from build123d import *

# Parameters (mm, degrees)
F1_DEPTH = 85
F3_DEPTH = 45
F5_DEPTH = 30
F6_SIZE2 = 20
F6_SIZE  = 68
F8_DEPTH = 30
F9_SIZE2 = 22
F9_SIZE  = 88


with BuildPart() as f1:
    # F0 (on Front) → F1 (new body)
    with BuildSketch(Plane.XZ):
        Polygon((-22.5, 0), (0, 0), (0, 2007.5), (785, 2007.5), (785, 0), (807.5, 0), (807.5, 2030), (-22.5, 2030), align=None)
    extrude(amount=F1_DEPTH)

    # F2 (on face) → F3 (join)
    with BuildSketch(Plane(origin=(0, 0, 0), x_dir=(-1, 0, 0), z_dir=(0, 1, 0))):
        Polygon((12.5, 0), (22.5, 0), (32.5, 0), (32.5, 2040), (-817.5, 2040), (-817.5, 0), (-807.5, 0), (-797.5, 0), (-797.5, 2020), (12.5, 2020), align=None)
    extrude(amount=F3_DEPTH)

    # F4 (on face) → F5 (join)
    with BuildSketch(Plane(origin=(0, 45, 0), x_dir=(-1, 0, 0), z_dir=(0, 1, 0))):
        Polygon((-897.5, 0), (-817.5, 0), (-807.5, 0), (-807.5, 2035), (27.5, 2035), (27.5, 0), (32.5, 0), (112.5, 0), (112.5, 2120), (-897.5, 2120), align=None)
    extrude(amount=F5_DEPTH)

    # F6
    f6_edges = [f1.edges().sort_by_distance(p)[0] for p in [
        (390, 75, 2035),
        (-27.5, 75, 1017.5),
        (807.5, 75, 1017.5),
    ]]
    f6_side = f1.faces().sort_by_distance((852.5, 75, 23.482973))[0]
    chamfer(f6_edges, length=F6_SIZE, length2=F6_SIZE2, reference=f6_side)

    # F7 (on face) → F8 (join)
    with BuildSketch(Plane.XZ.offset(85)):
        Polygon((-118, 0), (-8, 0), (-8, 2015.5), (793, 2015.5), (793, 0), (903, 0), (903, 2125.5), (-118, 2125.5), align=None)
    extrude(amount=F8_DEPTH)

    # F9
    f9_edges = [f1.edges().sort_by_distance(p)[0] for p in [
        (793, -115, 1007.75),
        (392.5, -115, 2015.5),
        (-8, -115, 1007.75),
    ]]
    f9_side = f1.faces().sort_by_distance((-63, -115, 23.580058))[0]
    chamfer(f9_edges, length=F9_SIZE, length2=F9_SIZE2, reference=f9_side)


solid = f1.part
Verification items for the finished model (mm, model axes). A direction names the side the tool comes from. Round coordinates to 2 decimals unless told otherwise and drop trailing zeros. Loops run counter-clockwise (first coordinate to the right, second up) from the corner with the lowest first, then second, coordinate; pieces in that order, holes last. Notation, with made-up numbers: (51, 32) - (60, 32) arc R15 ccw to (60, 47) - close; hole circle Ø10 at (-23, -22.75). An arc over 180 degrees is marked (long way). Write item = value, one per line.
Q1. Sectioned sample at B-B on x = 416. Record the boundary of the cut face in (y, z).
Here are the results:
outline = (-115, 2103.5) - (-93, 2015.5) - (-85, 2015.5) - (-85, 2007.5) - (0, 2007.5) - (0, 2020) - (45, 2020) - (45, 2035) - (55, 2035) - (75, 2103) - (75, 2120) - (45, 2120) - (45, 2040) - (0, 2040) - (0, 2030) - (-85, 2030) - (-85, 2125.5) - (-115, 2125.5) - close
Q2. Tool access check on faces 5 (the flat face through (844, 45, 1222)), 6 (the flat face through (387, -42, 2007.5)), 7 (the flat face through (-51.384, -103.846, 1037.026)), 8 (the flat face through (397, 65, 2069)), 9 (the flat face through (807.5, -42, 1001)). Record the directions out of +Z, -Z, +X, -X, +Y, -Y that give a thin tool (end or side, any length) a straight path to the whole face; none if there is none.
Here are the results:
face_5 = +Z
face_6 = -Z, +Y, -Y
face_7 = -Z, -Y
face_8 = -Z, +Y
face_9 = +Z, -Z, +X
Q3. Depth check by flat-ended pin: pin 1 (2 mm diameter, centred on x = 127, y = 26, fed in from +Z); pin 2 (6 mm diameter, centred on x = 28.5, y = -89.5, fed in from -Z); pin 3 (1 mm diameter, centred on y = -59, z = 251, fed in from +X). Enter the tip coordinate at first touch or a pass-through.
Here are the results:
pin_1 = 2040
pin_2 = 2015.5
pin_3 = 807.5
Q4. Material ranges on L1, parallel to X at y = -11, z = 2004.5; L2, parallel to X at y = 53.5, z = 381; L3, parallel to Y at x = 794, z = 340.5, recorded low to high.
Here are the results:
L1 = -22.5 to 0, 785 to 807.5
L2 = -112.5 to -27.5, 807.5 to 897.5
L3 = -93.25 to 0
Q5. Mould release check, pull along Y, two halves, no side actions. Record for faces 1 (the flat face through (387, 22, 2040)), 2 (the flat face through (-32.5, 22, 1006)), 3 (the flat face through (-61.02, 64.86, 1066.22)), 4 (the flat face through (804, -27, 0)): +Y half, -Y half, draft (parallel to the pull), parting line (faces both ways), or undercut.
Here are the results:
face_1 = undercut
face_2 = undercut
face_3 = +Y half
face_4 = draft
Q6. Sectioned sample at A-A on y = -34.5. Record the boundary of the cut face in (x, z).
Here are the results:
outline = (-22.5, 0) - (0, 0) - (0, 2007.5) - (785, 2007.5) - (785, 0) - (807.5, 0) - (807.5, 2030) - (-22.5, 2030) - close
